```python
from build123d import *

# Parameters (mm, degrees)
CROQUIS1_R              = 1.5
SALIENTE_EXTRUIR1_DEPTH = 2
CROQUIS2_R              = 3
CROQUIS2_R_2            = 1.5
SALIENTE_EXTRUIR3_DEPTH = 6
CORTAR_EXTRUIR2_START   = -6
CROQUIS4_R              = 1.5
CORTAR_EXTRUIR2_DEPTH   = 6


with BuildPart() as part:
    # Croquis1 → Saliente-Extruir1 (new body)
    with BuildSketch(Plane(origin=(0, 0, 0), x_dir=(1, 0, 0), z_dir=(0, 1, 0))):
        with BuildLine():
            Line((-17.320508076, 10), (17.320508076, 10))
            ThreePointArc((17.320508076, 10), (0, -20), (-17.320508076, 10))
        make_face()
        with Locations(Location((-16, -5.823523748, 0), (0, 0, 270))):
            Circle(CROQUIS1_R, mode=Mode.SUBTRACT)
        with Locations(Location((16, 5.823523748, 0), (0, 0, 270))):
            Circle(CROQUIS1_R, mode=Mode.SUBTRACT)
    extrude(amount=SALIENTE_EXTRUIR1_DEPTH)

    # Croquis2 → Saliente-Extruir3 (add)
    with BuildSketch(Plane(origin=(0, 0, 0), x_dir=(1, 0, 0), z_dir=(0, 1, 0))):
        with Locations(Location((0, 0, 0), (0, 0, 270))):
            Circle(CROQUIS2_R)
        with Locations(Location((0, 0, 0), (0, 0, 270))):
            Circle(CROQUIS2_R_2, mode=Mode.SUBTRACT)
    extrude(amount=-SALIENTE_EXTRUIR3_DEPTH)

    # Croquis4 → Cortar-Extruir2 (cut)
    with BuildSketch(Plane.XZ.offset(CORTAR_EXTRUIR2_START)):
        with Locations(Location((0, 0, 0), (0, 0, 90))):
            Circle(CROQUIS4_R)
    extrude(amount=CORTAR_EXTRUIR2_DEPTH, mode=Mode.SUBTRACT)


solid = part.part
```
The listing builds one solid part. Answer for the finished solid, in the listing's coordinates (mm). Round coordinates to 2 decimals unless told otherwise and drop trailing zeros. Order: outer loops, then holes, each group sorted by start corner. A loop starts at its lowest first (then second) coordinate and runs counter-clockwise, first axis right, second up. Notation, with made-up numbers: (63, 82.25) -> (105, 82.25) arc R27 cw to (105, 104.25) -> close; hole circle Ø3 at (-26.5, 84.25). An arc over 180 degrees is marked (long way). Answer as CSV lines item,"result".
Q1. A cutting plane is placed at C-C on x = -16.5. Determine the outline of the cut face in (y, z).
Computed values:
outline,"(0, -10) -> (2, -10) -> (2, 4.41) -> (0, 4.41) -> close; (0, 7.24) -> (2, 7.24) -> (2, 11.3) -> (0, 11.3) -> close"
Q2. A cutting plane is placed at B-B on y = 0.75. Determine the outline of the cut face in (x, z).
Computed values:
outline,"(-17.32, -10) -> (17.32, -10) arc R20 ccw (long way) to start; hole circle Ø3 at (-16, 5.82); hole circle Ø3 at (0, 0); hole circle Ø3 at (16, -5.82)"
Q3. For a pull along X with two mould halves and no side action, classify faces 1 (the cylindrical face through (-0.45, -1.94, 1.43)), 2 (the flat face through (0, 2, 5)), 3 (the cylindrical face through (16.451, 0.986, -4.393)), 4 (the cylindrical face through (0.9, -2.96, 2.86)) as +X half, -X half, draft (parallel to the pull), parting line (faces both ways), or undercut.
Computed values:
face 1,"undercut"
face 2,"draft"
face 3,"undercut"
face 4,"parting line"
Q4. Consider line 1 (X direction, y = -0.5, z = 0); line 2 (Y direction, x = 3, z = 7.25); line 3 (X direction, y = 1, z = -1.25). Determine where each line is inside the solid, lowest interval first. Write a range as from..to.
Computed values:
line 1,"x = -3..-1.5, 1.5..3"
line 2,"y = 0..2"
line 3,"x = -19.96..-0.83, 0.83..19.96"
Q5. A cutting plane is placed at A-A on x = 0. Determine the outline of the cut face in (y, z).
Computed values:
outline,"(-6, -3) -> (0, -3) -> (0, -10) -> (2, -10) -> (2, -1.5) -> (-6, -1.5) -> close; (-6, 1.5) -> (2, 1.5) -> (2, 20) -> (0, 20) -> (0, 3) -> (-6, 3) -> close"
Q6. A cutting plane is placed at D-D on y = -1.25. Determine the outline of the cut face in (x, z).
Computed values:
outline,"circle Ø6 at (0, 0); hole circle Ø3 at (0, 0)"
Q7. Given pin 1 (15 mm diameter, centred on x = 5, z = 9.5, fed in from -Y); pin 2 (4 mm diameter, centred on x = 0, z = 0, fed in from -Y); pin 3 (4 mm diameter, centred on x = 13.5, y = -3, fed in from -Z); pin 4 (4 mm diameter, centred on x = -3.5, y = -3.5, fed in from -Z), each flat-ended and moving along its own axis, determine where each tip first touches the part or whether it passes through.
Computed values:
pin 1,"stops at y = 0"
pin 2,"stops at y = -6"
pin 3,"passes through"
pin 4,"stops at z = -2.6"
